from build123d import *

# Parameters (mm, degrees)
F2_R = 1.27
F3_R = 0.635


with BuildPart() as f1:
    # F0 (on Front) → F1 (revolve)
    with BuildSketch(Plane.XZ):
        Polygon((-127, 0), (0, 0), (0, 12.7), (-50.8, 12.7), (-50.8, 19.05), (-76.2, 19.05), (-76.2, 25.4), (-127, 25.4), align=None)
    revolve(axis=Axis((-63.5, 0, 0), (-1, 0, 0)))

    # F2
    f2_edges = [f1.edges().sort_by_distance(p)[0] for p in [
        (0, 0, -12.7),
    ]]
    fillet(f2_edges, radius=F2_R)

    # F3
    f3_edges = [f1.edges().sort_by_distance(p)[0] for p in [
        (-50.8, 0, -19.05),
        (-76.2, 0, -25.4),
        (-127, 0, -25.4),
    ]]
    fillet(f3_edges, radius=F3_R)


solid = f1.part
Model file for the job. Use its own axes, mm. A direction names the side the tool comes from. Give positions to 0.01 mm unless a question says otherwise; leave off trailing zeros. Order: outer loops, then holes, each group sorted by start corner. A loop starts at its lowest first (then second) coordinate and runs counter-clockwise, first axis right, second up. Notation, with made-up numbers: M 22,-20 L 30,-20 A23 ccw 30,-11 Z; hole C -9,-38.5 d8. An arc over 180 degrees is marked long. Put each result on its own line as item: value. Start each with the question number.
(1) Band-saw the part on C-C on x = -20. Give the cut face in (y, z).
(2) Pin check, flat tips, straight feed: pin 1 Ø1 at (y, z) = (12, 20) entering from +X; pin 2 Ø2 at (x, y) = (-86.5, -9.5) entering from +Z; pin 3 Ø12 at (x, z) = (-111.5, 12) entering from -Y. Stop position of each tip, or through.
(3) Tool access for faces 1 (the face through (-127, 0, 0)), 2 (the face through (-63.99, -11.59, -15.12)): list every direction of +Z, -Z, +X, -X, +Y, -Y with a clear straight run to the whole face (end or side of a thin tool).
(4) Band-saw the part on A-A on z = 0. Give the cut face in (x, y) (3 decimals), then the cut area to 3 significant figures.
(5) Drill centre lines: L1, parallel to X at y = -19.5, z = 3.5; L2, parallel to X at y = 13, z = -12.5; L3, parallel to Z at x = -9, y = -0.5. Where is each one in solid material? Low to high. Write a range as [from, to].
Results below:
1. outline: C 0,0 d25.4
2. pin 1: stops at x = -76.2
2. pin 2: stops at z = 23.94
2. pin 3: stops at y = -24.68
3. face 1: +Z, -Z, -X, +Y, -Y
3. face 2: +X
4. outline: M -127,-24.765 A0.635 ccw -126.365,-25.4 L -76.835,-25.4 A0.635 ccw -76.2,-24.765 L -76.2,-19.05 L -51.435,-19.05 A0.635 ccw -50.8,-18.415 L -50.8,-12.7 L -1.27,-12.7 A1.27 ccw 0,-11.43 L 0,11.43 A1.27 ccw -1.27,12.7 L -50.8,12.7 L -50.8,18.415 A0.635 ccw -51.435,19.05 L -76.2,19.05 L -76.2,24.765 A0.635 ccw -76.835,25.4 L -126.365,25.4 A0.635 ccw -127,24.765 Z
4. area: 4,840 mm2
5. L1: x = [-127, -76.2]
5. L2: x = [-127, -50.8]
5. L3: z = [-12.69, 12.69]
